```python
from build123d import *

# Parameters (mm, degrees)
SKETCH1_R           = 2.25
BOSS_EXTRUDE1_DEPTH = 7.5
CUT_EXTRUDE1_START  = -7.5
SKETCH1_3_R         = 6.52
SKETCH1_3_R_2       = 2.25
CUT_EXTRUDE1_DEPTH  = 5
CUT_EXTRUDE2_START  = 2.5
SKETCH1_4_R         = 6.52
SKETCH1_4_R_2       = 2.25
CUT_EXTRUDE2_DEPTH  = 5
FILLET1_R           = 4
SKETCH2_R           = 2.1
CUT_EXTRUDE3_DEPTH  = 10
SKETCH3_W           = 7.5
SKETCH3_H           = 5.1
CUT_EXTRUDE4_DEPTH  = 37.510272694
CUT_EXTRUDE5_START  = -2.45
SKETCH2_7_R         = 2.1
CUT_EXTRUDE5_DEPTH  = 3


with BuildPart() as part:
    # Sketch1 → Boss-Extrude1 (new, symmetric)
    with BuildSketch(Plane.XY):
        with BuildLine():
            Line((0, 0), (0, 24))
            ThreePointArc((0, 24), (1.171572875, 26.828427125), (4, 28))
            Line((4, 28), (14, 28))
            ThreePointArc((14, 28), (16.828427125, 26.828427125), (18, 24))
            Line((18, 24), (18, 0))
            Line((18, 0), (0, 0))
        make_face()
        with Locations((9, 18)):
            Circle(SKETCH1_R, mode=Mode.SUBTRACT)
    extrude(amount=BOSS_EXTRUDE1_DEPTH, both=True)

    # Sketch1<3> → Cut-Extrude1 (cut)
    with BuildSketch(Plane.XY.offset(CUT_EXTRUDE1_START)):
        with Locations((9, 18)):
            Circle(SKETCH1_3_R)
        with Locations((9, 18)):
            Circle(SKETCH1_3_R_2, mode=Mode.SUBTRACT)
    extrude(amount=CUT_EXTRUDE1_DEPTH, mode=Mode.SUBTRACT)

    # Sketch1<4> → Cut-Extrude2 (cut)
    with BuildSketch(Plane.XY.offset(CUT_EXTRUDE2_START)):
        with Locations((9, 18)):
            Circle(SKETCH1_4_R)
        with Locations((9, 18)):
            Circle(SKETCH1_4_R_2, mode=Mode.SUBTRACT)
    extrude(amount=CUT_EXTRUDE2_DEPTH, mode=Mode.SUBTRACT)

    # Fillet1
    # the kernel refuses this fillet: 4 mm, written as the material it takes off along each edge
    with BuildSketch(Plane(origin=(4, 4, -3.5), x_dir=(0, -1, 0), z_dir=(-1, 0, 0))) as fillet1_piece_1_section:
        Polygon((0, 0), (FILLET1_R, 0), (FILLET1_R, -FILLET1_R), (0, -FILLET1_R), align=None)
    fillet1_piece_1 = extrude(amount=FILLET1_R, mode=Mode.PRIVATE)
    fillet1_piece_1 = fillet1_piece_1 - Plane(origin=(4, 4, -3.5), x_dir=(0, 0.7071067811865475, 0.7071067811865475), z_dir=(-1, 0, 0)) * Sphere(FILLET1_R, mode=Mode.PRIVATE)
    add(fillet1_piece_1, mode=Mode.SUBTRACT)
    with BuildSketch(Plane(origin=(4, 4, 3.5), x_dir=(0, -1, 0), z_dir=(-1, 0, 0))) as fillet1_piece_2_section:
        Polygon((0, 0), (FILLET1_R, 0), (FILLET1_R, FILLET1_R), (0, FILLET1_R), align=None)
    fillet1_piece_2 = extrude(amount=FILLET1_R, mode=Mode.PRIVATE)
    fillet1_piece_2 = fillet1_piece_2 - Plane(origin=(4, 4, 3.5), x_dir=(0, 0.7071067811865475, -0.7071067811865475), z_dir=(-1, 0, 0)) * Sphere(FILLET1_R, mode=Mode.PRIVATE)
    add(fillet1_piece_2, mode=Mode.SUBTRACT)
    with BuildSketch(Plane(origin=(14, 4, -3.5), x_dir=(0, 0, -1), z_dir=(0, -1, 0))) as fillet1_piece_3_section:
        Polygon((0, 0), (FILLET1_R, 0), (FILLET1_R, FILLET1_R), (0, FILLET1_R), align=None)
    fillet1_piece_3 = extrude(amount=FILLET1_R, mode=Mode.PRIVATE)
    fillet1_piece_3 = fillet1_piece_3 - Plane(origin=(14, 4, -3.5), x_dir=(-0.7071067811865475, 0, 0.7071067811865475), z_dir=(0, -1, 0)) * Sphere(FILLET1_R, mode=Mode.PRIVATE)
    add(fillet1_piece_3, mode=Mode.SUBTRACT)
    with BuildSketch(Plane(origin=(14, 4, 3.5), x_dir=(0, 0, 1), z_dir=(0, -1, 0))) as fillet1_piece_4_section:
        Polygon((0, 0), (FILLET1_R, 0), (FILLET1_R, -FILLET1_R), (0, -FILLET1_R), align=None)
    fillet1_piece_4 = extrude(amount=FILLET1_R, mode=Mode.PRIVATE)
    fillet1_piece_4 = fillet1_piece_4 - Plane(origin=(14, 4, 3.5), x_dir=(-0.7071067811865475, 0, -0.7071067811865475), z_dir=(0, -1, 0)) * Sphere(FILLET1_R, mode=Mode.PRIVATE)
    add(fillet1_piece_4, mode=Mode.SUBTRACT)
    with BuildSketch(Plane(origin=(0, 4, -7.5), x_dir=(0, 0, 1), z_dir=(0, 1, 0)), Plane(origin=(18, 24, 7.5), x_dir=(-1, 0, 0), z_dir=(0, -1, 0))) as fillet1_piece_5:
        with BuildLine():
            CenterArc((FILLET1_R, FILLET1_R), FILLET1_R, 180, 90)
            Line((0, FILLET1_R), (0, 0))
            Line((0, 0), (FILLET1_R, 0))
        make_face()
    extrude(amount=20, mode=Mode.SUBTRACT)
    with BuildSketch(Plane(origin=(4, 24, -7.5), x_dir=(-1, 0, 0), z_dir=(0, -1, 0))) as fillet1_piece_6:
        with BuildLine():
            CenterArc((4 - FILLET1_R, -FILLET1_R), FILLET1_R, 0, 90)
            Line((4, -FILLET1_R), (4, 0))
            Line((4, 0), (4 - FILLET1_R, 0))
        make_face()
    revolve(axis=Axis((4, 24, -7.5), (0, 0, -1)), revolution_arc=90, mode=Mode.SUBTRACT)
    with BuildSketch(Plane(origin=(0, 4, 7.5), x_dir=(0, 0, -1), z_dir=(0, 1, 0)), Plane(origin=(18, 24, -7.5), x_dir=(-1, 0, 0), z_dir=(0, -1, 0))) as fillet1_piece_7:
        with BuildLine():
            CenterArc((FILLET1_R, -FILLET1_R), FILLET1_R, 90, 90)
            Line((0, -FILLET1_R), (0, 0))
            Line((0, 0), (FILLET1_R, 0))
        make_face()
    extrude(amount=20, mode=Mode.SUBTRACT)
    with BuildSketch(Plane(origin=(18, 0, -3.5), x_dir=(-1, 0, 0), z_dir=(0, 0, 1)), Plane(origin=(0, 0, -3.5), x_dir=(0, 1, 0), z_dir=(0, 0, 1))) as fillet1_piece_8:
        with BuildLine():
            CenterArc((FILLET1_R, -FILLET1_R), FILLET1_R, 90, 90)
            Line((0, -FILLET1_R), (0, 0))
            Line((0, 0), (FILLET1_R, 0))
        make_face()
    extrude(amount=7, mode=Mode.SUBTRACT)
    with BuildSketch(Plane(origin=(14, 0, 7.5), x_dir=(0, 0, -1), z_dir=(-1, 0, 0)), Plane(origin=(4, 28, -7.5), x_dir=(0, -1, 0), z_dir=(1, 0, 0))) as fillet1_piece_9:
        with BuildLine():
            CenterArc((FILLET1_R, -FILLET1_R), FILLET1_R, 90, 90)
            Line((0, -FILLET1_R), (0, 0))
            Line((0, 0), (FILLET1_R, 0))
        make_face()
    extrude(amount=10, mode=Mode.SUBTRACT)
    with BuildSketch(Plane(origin=(14, 24, 7.5), x_dir=(0, 1, 0), z_dir=(-1, 0, 0))) as fillet1_piece_10:
        with BuildLine():
            CenterArc((4 - FILLET1_R, FILLET1_R), FILLET1_R, 270, 90)
            Line((4, FILLET1_R), (4, 0))
            Line((4, 0), (4 - FILLET1_R, 0))
        make_face()
    revolve(axis=Axis((14, 24, 7.5), (0, 0, -1)), revolution_arc=90, mode=Mode.SUBTRACT)
    with BuildSketch(Plane(origin=(4, 28, 7.5), x_dir=(0, -1, 0), z_dir=(1, 0, 0)), Plane(origin=(14, 0, -7.5), x_dir=(0, 0, 1), z_dir=(-1, 0, 0))) as fillet1_piece_11:
        with BuildLine():
            CenterArc((FILLET1_R, FILLET1_R), FILLET1_R, 180, 90)
            Line((0, FILLET1_R), (0, 0))
            Line((0, 0), (FILLET1_R, 0))
        make_face()
    extrude(amount=10, mode=Mode.SUBTRACT)
    with BuildSketch(Plane(origin=(14, 24, -7.5), x_dir=(0, 1, 0), z_dir=(-1, 0, 0))) as fillet1_piece_12:
        with BuildLine():
            CenterArc((4 - FILLET1_R, -FILLET1_R), FILLET1_R, 0, 90)
            Line((4, -FILLET1_R), (4, 0))
            Line((4, 0), (4 - FILLET1_R, 0))
        make_face()
    revolve(axis=Axis((14, 24, -7.5), (0, 0, -1)), revolution_arc=90, mode=Mode.SUBTRACT)
    with BuildSketch(Plane(origin=(4, 24, 7.5), x_dir=(-1, 0, 0), z_dir=(0, -1, 0))) as fillet1_piece_13:
        with BuildLine():
            CenterArc((4 - FILLET1_R, FILLET1_R), FILLET1_R, 270, 90)
            Line((4 - FILLET1_R, 0), (4, 0))
            Line((4, 0), (4, FILLET1_R))
        make_face()
    revolve(axis=Axis((4, 24, 7.5), (0, 0, -1)), revolution_arc=90, mode=Mode.SUBTRACT)

    # Sketch2 → Cut-Extrude3 (cut)
    with BuildSketch(Plane.XZ):
        with Locations((9, 0)):
            Circle(SKETCH2_R)
    extrude(amount=-CUT_EXTRUDE3_DEPTH, mode=Mode.SUBTRACT)

    # Sketch3 → Cut-Extrude4 (cut, through all)
    with BuildSketch(Plane(origin=(0, 0, -7.5), x_dir=(-1, 0, 0), z_dir=(0, 0, -1))):
        with Locations((-9, 8)):
            Rectangle(SKETCH3_W, SKETCH3_H)
    extrude(amount=-CUT_EXTRUDE4_DEPTH, mode=Mode.SUBTRACT)

    # Sketch2<7> → Cut-Extrude5 (cut)
    with BuildSketch(Plane.XZ.offset(CUT_EXTRUDE5_START)):
        Polygon((12.461165772, -2.005076432), (12.467030013, 1.994919269), (9.005864241, 3.999995701), (5.538834228, 2.005076432), (5.532969987, -1.994919269), (8.994135759, -3.999995701), align=None)
        with Locations((9, 0)):
            Circle(SKETCH2_7_R, mode=Mode.SUBTRACT)
    extrude(amount=-CUT_EXTRUDE5_DEPTH, mode=Mode.SUBTRACT)


solid = part.part
```
Work out the finished part from the listing and answer in its coordinate system (mm). A direction names the side the tool comes from. Round coordinates to 2 decimals unless told otherwise and drop trailing zeros. Write each loop counter-clockwise with the first axis right and the second up, starting at its lowest first coordinate (ties: lowest second). Pieces come first, ordered by that corner, then holes. Notation, with made-up numbers: (0, -35) -> (27, -35) arc R27 cw to (27, -2) -> close; hole circle Ø2 at (15, 47.25). An arc over 180 degrees is marked (long way). Write each question's results on one line, items separated by ' | '.
1) Consider line 1 along Y through (x, z) = (14, 3); line 2 along Y through (x, z) = (9, -4.2); line 3 along Y through (x, z) = (9, 5.3). Determine where each line is inside the solid, lowest interval first. Write a range as [from, to].
Findings:
line 1: y = [0, 13.82], [22.18, 28] | line 2: y = [0.06, 5.45], [10.55, 11.48], [24.52, 27.94] | line 3: y = [0.43, 5.45], [10.55, 11.48], [24.52, 27.57]
2) The part is cut by section A-A (y = 8). Write down the section's boundary in (x, z), and give its area (3 significant figures).
Findings:
outline: (0, -3.5) arc R4 ccw to (4, -7.5) -> (5.25, -7.5) -> (5.25, 7.5) -> (4, 7.5) arc R4 ccw to (0, 3.5) -> close; (12.75, -7.5) -> (14, -7.5) arc R4 ccw to (18, -3.5) -> (18, 3.5) arc R4 ccw to (14, 7.5) -> (12.75, 7.5) -> close | area: 144 mm²
3) The part is cut by section C-C (x = 8.5). State how many separate pieces and enclosed holes the cut face has, and give its area (3 significant figures).
Findings:
separate pieces: 4 | enclosed holes: 0 | area: 146 mm²
4) For a pull along Y with two mould halves and no side action, classify faces 1 (the flat face through (7.3, 3.93, 3.02)), 2 (the cylindrical face through (1.141, 26.797, 0.049)), 3 (the flat face through (0, 14, 0)) as +Y half, -Y half, draft (parallel to the pull), parting line (faces both ways), or undercut.
Findings:
face 1: undercut | face 2: +Y half | face 3: draft
5) The part is cut by section D-D (z = 1.25). Write down the section's boundary in (x, y), and give its area (3 significant figures).
Findings:
outline: (0, 4) arc R4 ccw to (4, 0) -> (7.31, 0) -> (7.31, 2.45) -> (5.54, 2.45) -> (5.54, 5.45) -> (5.25, 5.45) -> (5.25, 10.55) -> (12.75, 10.55) -> (12.75, 5.45) -> (12.47, 5.45) -> (12.47, 2.45) -> (10.69, 2.45) -> (10.69, 0) -> (14, 0) arc R4 ccw to (18, 4) -> (18, 24) arc R4 ccw to (14, 28) -> (4, 28) arc R4 ccw to (0, 24) -> close; hole circle Ø4.5 at (9, 18) | area: 407 mm²
6) The part is cut by section B-B (z = 5.5). Write down the section's boundary in (x, y), and give its area (3 significant figures).
Findings:
outline: (0.54, 4) arc R3.46 ccw to (4, 0.54) -> (14, 0.54) arc R3.46 ccw to (17.46, 4) -> (17.46, 24) arc R3.46 ccw to (14, 27.46) -> (4, 27.46) arc R3.46 ccw to (0.54, 24) -> close; hole circle Ø13.04 at (9, 18); hole (5.25, 5.45) -> (12.75, 5.45) -> (12.75, 10.55) -> (5.25, 10.55) -> close | area: 274 mm²
7) Which of the six approach directions +Z, -Z, +X, -X, +Y, -Y give full straight-line access (tool end or side, diameter ignored) to faces 4 (the cylindrical face through (9.07, 1.203, -6.359)), 5 (the flat face through (9, 15, -2.5)), 6 (the cylindrical face through (16.859, 14.14, 6.297)), 7 (the flat face through (10.7, 5.45, -3.4)), 8 (the flat face through (10.761, 3.929, 2.983))?
Findings:
face 4: -Z, +X, -X, -Y | face 5: -Z | face 6: +Z, +X, +Y, -Y | face 7: +Z, -Z | face 8: none
8) Flat-ended cylindrical pins translate along their axes: pin 1 (3 mm diameter, centred on x = 10.5, y = 19, fed in from -Z); pin 2 (6.5 mm diameter, centred on x = 6, y = 16.5, fed in from +Z); pin 3 (1.5 mm diameter, centred on x = 7.5, y = 21.5, fed in from +Z). Find the tip coordinate at first contact, or state that the pin passes through.
Findings:
pin 1: stops at z = -2.5 | pin 2: stops at z = 7.49 | pin 3: stops at z = 2.5
